```python
from build123d import *

# Parameters (mm, degrees)
F0_R     = 29.21
F0_R_2   = 8.4188415788
F1_DEPTH = 1.524
F0_R_3   = 6.35
F2_DEPTH = 24.638
F3_R     = 3.3954821981
F4_DEPTH = 8.382


with BuildPart() as f1:
    # F0 (on Front) → F1 (new body)
    with BuildSketch(Plane.XZ):
        Circle(F0_R)
        Circle(F0_R_2, mode=Mode.SUBTRACT)
    extrude(amount=F1_DEPTH)

    # F0 (on Front) → F2 (join)
    with BuildSketch(Plane.XZ):
        Circle(F0_R_2)
        Circle(F0_R_3, mode=Mode.SUBTRACT)
    extrude(amount=F2_DEPTH)

    # F3 (on face) → F4 (join)
    with BuildSketch(Plane(origin=(0, 0, 0), x_dir=(-1, 0, 0), z_dir=(0, 1, 0))):
        with Locations((8.4494473413, 21.9940822572)):
            Circle(F3_R)
    extrude(amount=F4_DEPTH)


solid = f1.part
```
Check sheet for the modelled part. Datum: model origin and axes. Units: mm. A direction names the side the tool comes from. Round coordinates to 2 decimals unless told otherwise and drop trailing zeros. Order: outer loops, then holes, each group sorted by start corner. A loop starts at its lowest first (then second) coordinate and runs counter-clockwise, first axis right, second up.
1) Section check A-A (z = 0). Record the boundary of the cut face in (x, y).
2) Section check B-B (x = 0). Record the boundary of the cut face in (y, z).
3) Go/stop test with flat-tipped pins: pin 1 Ø6 at (y, z) = (-20, -10.5) entering from +X; pin 2 Ø4 at (x, y) = (4, -20) entering from +Z; pin 3 Ø12 at (x, z) = (-2, -6.5) entering from +Y. Record where each tip stops, or that it passes through.
4) Mould release check, pull along X, two halves, no side actions. Record for faces 1 (the cylindrical face through (-21.53, -0.75, 19.74)), 2 (the cylindrical face through (-1.38, -12.15, -6.2)), 3 (the flat face through (-3, -24.638, 6)): +X half, -X half, draft (parallel to the pull), parting line (faces both ways), or undercut.
5) Scan lines: line 1 (Z direction, x = 0, y = -19); line 2 (Y direction, x = -8.5, z = -9); line 3 (X direction, y = -17.5, z = 3). Record each from-to range of solid material in increasing order.
6) Section check C-C (y = -19). Record the boundary of the cut face in (x, z), and give its area (3 significant figures).
7) Section check D-D (z = 20). Record the boundary of the cut face in (x, y).
8) Tool access check on faces 4 (the cylindrical face through (-8.01, 4.13, 25.36)), 5 (the cylindrical face through (-8.41, -12.92, 0.37)), 6 (the flat face through (-8, 8.382, 22)). Record the directions out of +Z, -Z, +X, -X, +Y, -Y that give a thin tool (end or side, any length) a straight path to the whole face; none if there is none.
Result:
1. outline: (-29.21, -1.52) - (-8.42, -1.52) - (-8.42, -24.64) - (-6.35, -24.64) - (-6.35, 0) - (-29.21, 0) - close; (6.35, -24.64) - (8.42, -24.64) - (8.42, -1.52) - (29.21, -1.52) - (29.21, 0) - (6.35, 0) - close
2. outline: (-24.64, -8.42) - (-1.52, -8.42) - (-1.52, -29.21) - (0, -29.21) - (0, -6.35) - (-24.64, -6.35) - close; (-24.64, 6.35) - (0, 6.35) - (0, 29.21) - (-1.52, 29.21) - (-1.52, 8.42) - (-24.64, 8.42) - close
3. pin 1: stops at x = 3.82
3. pin 2: stops at z = 8.18
3. pin 3: stops at y = 0
4. face 1: parting line
4. face 2: undercut
4. face 3: draft
5. line 1: z = -8.42 to -6.35, 6.35 to 8.42
5. line 2: y = -1.52 to 0
5. line 3: x = -7.87 to -5.6, 5.6 to 7.87
6. outline: circle Ø16.84 at (0, 0); hole circle Ø12.7 at (0, 0)
6. area: 96.0 mm2
7. outline: (-21.29, -1.52) - (21.29, -1.52) - (21.29, 0) - (-5.7, 0) - (-5.7, 8.38) - (-11.2, 8.38) - (-11.2, 0) - (-21.29, 0) - close
8. face 4: +Y
8. face 5: -Y
8. face 6: +Z, -Z, +X, -X, +Y
